```python
from build123d import *

# Parameters (mm, degrees)
F0_R     = 4.5
F0_R_2   = 5.1
F1_DEPTH = 8


with BuildPart() as f1:
    # F0 (on Front) → F1 (new body)
    with BuildSketch(Plane.XZ):
        with BuildLine():
            Line((0, -38), (0, 0))
            Line((0, 0), (-45, 0))
            Line((-45, 0), (-45, -30))
            Line((-45, -30), (-38, -30))
            ThreePointArc((-38, -30), (-34.464466, -31.464466), (-33, -35))
            Line((-33, -35), (-33, -80))
            Line((-33, -80), (-7.6, -80))
            Line((-7.6, -80), (-7.6, -60))
            Line((-7.6, -60), (-16, -60))
            ThreePointArc((-16, -60), (-17.414214, -59.414214), (-18, -58))
            Line((-18, -58), (-18, -40))
            ThreePointArc((-18, -40), (-17.414214, -38.585786), (-16, -38))
            Line((-16, -38), (0, -38))
        make_face()
        with Locations((-22, -69.5)):
            Circle(F0_R, mode=Mode.SUBTRACT)
        with Locations((-25, -15)):
            Circle(F0_R_2, mode=Mode.SUBTRACT)
    extrude(amount=F1_DEPTH)

    # F2: F1 across face


with BuildPart() as f1_1:
    add(f1.part)
    add(f1.part.mirror(Plane(origin=(0, -4, -19), x_dir=(0, 1, 0), z_dir=(1, 0, 0))))


solid = f1_1.part
```
Geometry check sheet. Reference: the model listing, model coordinates, mm. A direction names the side the tool comes from. Coordinates: 2 decimals unless noted, no trailing zeros. Order: outer loops, then holes, each group sorted by start corner. A loop starts at its lowest first (then second) coordinate and runs counter-clockwise, first axis right, second up.
Q1. Sectioned sample at D-D on z = -69.5. Record the cut outline in (x, y).
Reply:
outline: (-33, -8) - (-26.5, -8) - (-26.5, 0) - (-33, 0) - close; (-17.5, -8) - (-7.6, -8) - (-7.6, 0) - (-17.5, 0) - close; (7.6, -8) - (17.5, -8) - (17.5, 0) - (7.6, 0) - close; (26.5, -8) - (33, -8) - (33, 0) - (26.5, 0) - close
Q2. Sectioned sample at B-B on y = -6.5. Record the cut outline in (x, z), and give its area (3 significant figures).
Reply:
outline: (-45, -30) - (-38, -30) arc R5 cw to (-33, -35) - (-33, -80) - (-7.6, -80) - (-7.6, -60) - (-16, -60) arc R2 cw to (-18, -58) - (-18, -40) arc R2 cw to (-16, -38) - (16, -38) arc R2 cw to (18, -40) - (18, -58) arc R2 cw to (16, -60) - (7.6, -60) - (7.6, -80) - (33, -80) - (33, -35) arc R5 cw to (38, -30) - (45, -30) - (45, 0) - (-45, 0) - close; hole circle Ø10.2 at (-25, -15); hole circle Ø9 at (-22, -69.5); hole circle Ø9 at (22, -69.5); hole circle Ø10.2 at (25, -15)
area: 4,630 mm2
Q3. Depth check by flat-ended pin: pin 1 Ø1.5 at (y, z) = (-2, -65.5) entering from +X; pin 2 Ø1.5 at (y, z) = (-2.5, -53.5) entering from -X; pin 3 Ø2 at (x, y) = (41.5, -2) entering from -Z. Enter the tip coordinate at first touch or a pass-through.
Reply:
pin 1: stops at x = 33
pin 2: stops at x = -33
pin 3: stops at z = -30
Q4. Tool access check on faces 1 (the face through (-45, -4, -15)), 2 (the face through (45, -4, -15)), 3 (the face through (-33, -4, -57)), 4 (the face through (7.6, -4, -70)), 5 (the face through (-17.43, -3.94, -38.6)). Record the directions out of +Z, -Z, +X, -X, +Y, -Y that give a thin tool (end or side, any length) a straight path to the whole face; none if there is none.
Reply:
face 1: +Z, -Z, -X, +Y, -Y
face 2: +Z, -Z, +X, +Y, -Y
face 3: -Z, -X, +Y, -Y
face 4: -Z, +Y, -Y
face 5: +Y, -Y
Q5. Thickness scan on probe 1 along X at (y, z) = (-2, -54.5); probe 2 along X at (y, z) = (-4.25, -66); probe 3 along X at (y, z) = (-2, -77). Record the ranges inside material, lowest first.
Reply:
probe 1: x = -33 to -18, 18 to 33
probe 2: x = -33 to -24.83, -19.17 to -7.6, 7.6 to 19.17, 24.83 to 33
probe 3: x = -33 to -7.6, 7.6 to 33
Q6. Sectioned sample at A-A on z = -15. Record the cut outline in (x, y).
Reply:
outline: (-45, -8) - (-30.1, -8) - (-30.1, 0) - (-45, 0) - close; (-19.9, -8) - (19.9, -8) - (19.9, 0) - (-19.9, 0) - close; (30.1, -8) - (45, -8) - (45, 0) - (30.1, 0) - close
Q7. Sectioned sample at C-C on x = 12.5. Record the cut outline in (y, z), and give its area (3 significant figures).
Reply:
outline: (-8, -80) - (0, -80) - (0, -60) - (-8, -60) - close; (-8, -38) - (0, -38) - (0, 0) - (-8, 0) - close
area: 464 mm2
Q8. Draft check along X on faces 6 (the face through (-35, -4, -31)), 7 (the face through (17.4, -3.94, -59.43)), 8 (the face through (1, 0, -31)), 9 (the face through (35, -4, -31)). Enter one of: released by +X, released by -X, zero draft, split by the parting line, or undercut.
Reply:
face 6: released by -X
face 7: undercut
face 8: zero draft
face 9: released by +X
